Can you work these out from the model? Positions are in its coordinate system, mm. Face numbers are marked on the shaded views. A direction names the side the tool comes from. Round coordinates to 2 decimals unless told otherwise and drop trailing zeros. Loops run counter-clockwise (first coordinate to the right, second up) from the corner with the lowest first, then second, coordinate; pieces in that order, holes last. Notation, with made-up numbers: (56, 10) -> (74, 10) arc R25 ccw to (74, 46) -> close; hole circle Ø11 at (77, 0.25). An arc over 180 degrees is marked (long way). Answer as a JSON object with one key per item and string values.
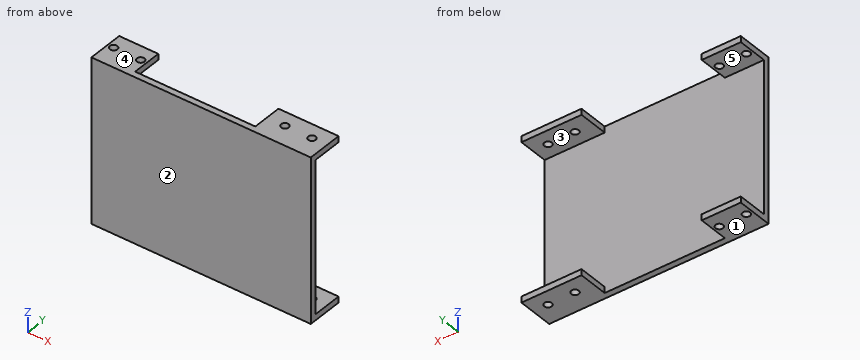
```python
from build123d import *

# Parameters (mm, degrees)
SKETCH1_W           = 73
SKETCH1_H           = 54.5
BOSS_EXTRUDE1_DEPTH = 2
SKETCH2_W           = 20
SKETCH2_H           = 2
SKETCH2_W_2         = 13
BOSS_EXTRUDE2_DEPTH = 10
SKETCH3_R           = 1.25
CUT_EXTRUDE1_DEPTH  = 55.5


with BuildPart() as part:
    # Sketch1 → Boss-Extrude1 (new body)
    with BuildSketch(Plane(origin=(0, 0, 0), x_dir=(1, 0, 0), z_dir=(0, 1, 0))):
        with Locations((-15.498549405, 1.944031796)):
            Rectangle(SKETCH1_W, SKETCH1_H)
    extrude(amount=BOSS_EXTRUDE1_DEPTH)

    # Sketch2 → Boss-Extrude2 (add)
    with BuildSketch(Plane(origin=(0, 2, 0), x_dir=(1, 0, 0), z_dir=(0, 1, 0))):
        with Locations((11.001450595, 28.194031796)):
            Rectangle(SKETCH2_W, SKETCH2_H)
        with Locations((11.001450595, -24.305968204)):
            Rectangle(SKETCH2_W, SKETCH2_H)
        with Locations((-45.498549405, 28.194031796)):
            Rectangle(SKETCH2_W_2, SKETCH2_H)
        with Locations((-45.498549405, -24.305968204)):
            Rectangle(SKETCH2_W_2, SKETCH2_H)
    extrude(amount=BOSS_EXTRUDE2_DEPTH)

    # Sketch3 → Cut-Extrude1 (cut, through all)
    with BuildSketch(Plane.XY.offset(25.305968204)):
        with Locations((16.001450595, 7)):
            Circle(SKETCH3_R)
        with Locations((7.001450595, 7)):
            Circle(SKETCH3_R)
        with Locations((-40.998549405, 7)):
            Circle(SKETCH3_R)
        with Locations((-49.998549405, 7)):
            Circle(SKETCH3_R)
    extrude(amount=-CUT_EXTRUDE1_DEPTH, mode=Mode.SUBTRACT)


solid = part.part
```
Q1. I want a section at A-A, the plane y = 3. Write out the boundary of the cut face in (x, z).
Determined:
{"outline": "(-52, -29.19) -> (-39, -29.19) -> (-39, -27.19) -> (-52, -27.19) -> close; (-52, 23.31) -> (-39, 23.31) -> (-39, 25.31) -> (-52, 25.31) -> close; (1, -29.19) -> (21, -29.19) -> (21, -27.19) -> (1, -27.19) -> close; (1, 23.31) -> (21, 23.31) -> (21, 25.31) -> (1, 25.31) -> close"}
Q2. We'd pull the mould along Z, two halves only. Please class the marked faces 1, 2 and 3: pulls with the +Z half, pulls with the -Z half, needs draft (parallel to the pull), parting line crosses it, or undercut.
Determined:
{"face 1": "pulls with the -Z half", "face 2": "needs draft", "face 3": "undercut"}
Q3. I want a section at C-C, the plane y = 7. Give the number of separate pieces and of enclosed holes in the cut face, then the cut area to 3 significant figures.
Determined:
{"separate pieces": "12", "enclosed holes": "0", "area": "92.0 mm²"}
Q4. On a 3-axis mill with a long thin cutter (end or side, diameter ignored), from which of +Z, -Z, +X, -X, +Y, -Y can I reach the whole of each face in a straight line? I mean the marked faces 4 and 5. Say none if no direction works.
Determined:
{"face 4": "+Z, +X, -X, +Y, -Y", "face 5": "+X, -X, +Y"}
Q5. I want a section at B-B, the plane x = 15.5. Write out the boundary of the cut face in (y, z) (3 decimals), then the cut area to 3 significant figures.
Determined:
{"outline": "(0, -29.194) -> (5.855, -29.194) -> (5.855, -27.194) -> (2, -27.194) -> (2, 23.306) -> (5.855, 23.306) -> (5.855, 25.306) -> (0, 25.306) -> close; (8.145, -29.194) -> (12, -29.194) -> (12, -27.194) -> (8.145, -27.194) -> close; (8.145, 23.306) -> (12, 23.306) -> (12, 25.306) -> (8.145, 25.306) -> close", "area": "140 mm²"}
Q6. If I drill on L1, parallel to X at y = 8.75, z = 23.5; L2, parallel to Z at x = 5, y = 10.75; L3, parallel to Y at x = -38.5, z = 18, over which ranges is the centre line in solid material (lowest first)? Write a range as [from, to].
Determined:
{"L1": "[-52, -39], [1, 21]", "L2": "[-29.19, -27.19], [23.31, 25.31]", "L3": "[0, 2]"}
Q7. I want a section at D-D, the plane x = -3.5. Write out the boundary of the cut face in (y, z).
Determined:
{"outline": "(0, -29.19) -> (2, -29.19) -> (2, 25.31) -> (0, 25.31) -> close"}
